Input: part model. Units: mm. Frame: model coordinates. A direction names the side the tool comes from. Round coordinates to 2 decimals unless told otherwise and drop trailing zeros. Loops run counter-clockwise (first coordinate to the right, second up) from the corner with the lowest first, then second, coordinate; pieces in that order, holes last. Notation, with made-up numbers: M 49,64 L 77,64 A25 ccw 77,76 Z; hole C 73.25,-23.5 d3. An arc over 180 degrees is marked long. Put each result on its own line as item: value. Start each with the question number.
1) Reachability of faces 5 (the face through (15, 5, 31.5)), 6 (the face through (-7, 14, 34.5)), 7 (the face through (0, 10, 0)) from +Z, -Z, +X, -X, +Y, -Y: full face, straight path, thin tool, end or side. Return the list, or none.
2) Section D-D on z = 37. Output: boundary loops of the cut face in (x, y), plus the area to 3 significant figures.
3) Line query: probe 1 along Z at (x, y) = (-7, 4.5); probe 2 along Y at (x, z) = (-7.08, 36.75); probe 3 along Z at (x, y) = (7.8, 2). Output: solid intervals per line, ascending.
4) Draft query along Z for faces 1 (the face through (-7, 10, 41.5)), 2 (the face through (-7, 20, 37)), 3 (the face through (8.421, 4.93, 15.797)), 4 (the face through (-7.487, 4.93, -16.954)). Return one class per face: +Z half, -Z half, draft (parallel to the pull), parting line (faces both ways), or undercut.
5) Pin query (flat end, axial travel): pin 1 (2.5 mm diameter, centred on x = -7, z = 23.5, fed in from -Y); pin 2 (1 mm diameter, centred on x = -11.5, z = 30, fed in from +Y); pin 3 (1.5 mm diameter, centred on x = 12.5, y = 5, fed in from +Z); pin 4 (8 mm diameter, centred on y = 3, z = 5, fed in from -X). Return the tip coordinate at first contact, or that it passes through.
6) Section B-B on z = 23.5. Output: boundary loops of the cut face in (x, y).
7) Section C-C on x = -11.5. Output: boundary loops of the cut face in (y, z), plus the area to 3 significant figures.
8) Section A-A on y = 4. Output: boundary loops of the cut face in (x, z), plus the area to 3 significant figures.
Autodesk Inventor part; units mm, degrees
ref_plane "YZ Plane" through (0, 0, 0) normal (1, 0, 0) x (0, 1, 0)
ref_plane "XZ Plane" through (0, 0, 0) normal (0, 1, 0) x (-1, 0, 0)
ref_plane "XY Plane" through (0, 0, 0) normal (0, 0, 1) x (1, 0, 0)
sketch "Sketch2" plane through (0, 0, 0) normal (0, 1, 0) x (-1, 0, 0)
  line L0 (0, -46.1) -> (0, 56.1)
  line L1 (33.556, 0) -> (-28.926, 0)
  line L2 (20, -31.5) -> (-20, -31.5)
  line L3 (-20, -31.5) -> (-20, 31.5)
  line L4 (-20, 31.5) -> (20, 31.5)
  line L5 (20, 31.5) -> (20, -31.5)
  line L6 (20, -31.5) -> (-20, 31.5) construction
  line L7 (-20, -31.5) -> (20, 31.5) construction
  line L8 (24.63, 31.5) -> (-10.47, 31.5)
  line L9 (-10.47, 31.5) -> (-10.47, 41.5)
  line L10 (-10.47, 41.5) -> (24.63, 41.5)
  line L11 (24.63, 41.5) -> (24.63, 31.5)
  line L12 (24.63, 31.5) -> (-10.47, 41.5) construction
  line L13 (-10.47, 31.5) -> (24.63, 41.5) construction
  point P0 (0, 0)
  point P1 (7.08, 36.5)
  point P2 (-10.47, 31.5)
  dimension "d5" = 40
  dimension "d6" = 63
  dimension "d7" = 9.53
  dimension "d8" = 35.1
  dimension "d9" = 73
extrude "Extrusion1" add sketch "Sketch2" along normal blind 10 contours L2 L3 L1 L0 | L0 L1 L5 L2 | L1 L3 L4 L0 | L0 L4 L5 L1
extrude "Extrusion2" add sketch "Sketch2" along normal blind 20 contours L4 L9 L10 L0 | L0 L10 L11 L8 L4
sketch "Sketch3" plane through (0, 10, 0) normal (0, 1, 0) x (1, 0, 0)
  line L0 (-20, 31.5) -> (-20, -31.5)
  line L1 (20, 31.5) -> (-20, 31.5)
  line L2 (20, -31.5) -> (20, 31.5)
  point P0 (0, 0)
  point P1 (-7, 18.5)
  point P2 (-7, -23.5)
  point P3 (7.8, 14.41)
  point P4 (7.8, -14.3)
  dimension "d21" = 13
  dimension "d22" = 13
  dimension "d23" = 42
  dimension "d24" = 13
  dimension "d25" = 12.2
  dimension "d26" = 12.2
  dimension "d27" = 17.09
  dimension "d28" = 28.71
hole "Hole1" at (-7, 10, -18.5) at (-7, 10, 23.5) at (7.8, 10, -14.41) at (7.8, 10, 14.3) direction (0, -1, 0) diameter 3.242 end through all
sketch "Sketch4" plane through (-24.63, 0, 41.5) normal (0, 0, 1) x (1, 0, 0)
  line L0 (0, 20) -> (35.1, 20)
  line L1 (35.1, 0) -> (35.1, 20)
  point P0 (24.63, 0)
  point P1 (17.55, 14.3)
  dimension "d36" = 5.7
  dimension "d37" = 17.55
hole "Hole2" at (-7.08, 14.3, 41.5) direction (0, 0, -1) diameter 7.4 depth 7
sketch "Sketch5" plane through (-24.63, 0, 41.5) normal (0, 0, 1) x (1, 0, 0)
  circle A0 centre (17.55, 14.3) radius 3.7
  line L0 (0, 0) -> (35.1, 0)
  line L1 (35.1, 0) -> (35.1, 20)
  point P0 (24.63, 0)
  point P1 (17.55, 4)
  dimension "d46" = 4
  dimension "d47" = 17.55
hole "Hole3" at (-7.08, 4, 41.5) direction (0, 0, -1) diameter 4 depth 7
properties part number "uchwyt_strzykawka_dol" material "PC/ABS Plastic"
Geometry results:
1. face 5: +Z, +X, +Y, -Y
1. face 6: +Z
1. face 7: -Z, +X, -X, +Y
2. outline: M -24.63,0 L 10.47,0 L 10.47,20 L -24.63,20 Z; hole C -7.08,14.3 d7.4; hole C -7.08,4 d4
2. area: 646 mm²
3. probe 1: z = -31.5 to -20.12, -16.88 to 21.88, 25.12 to 34.5
3. probe 2: y = 0 to 2, 6 to 10.6, 18 to 20
3. probe 3: z = -31.5 to -16.03, -12.79 to 12.68, 15.92 to 41.5
4. face 1: +Z half
4. face 2: draft
4. face 3: undercut
4. face 4: undercut
5. pin 1: passes through
5. pin 2: stops at y = 10
5. pin 3: stops at z = 31.5
5. pin 4: stops at x = -20
6. outline: M -20,0 L -8.62,0 L -8.62,10 L -20,10 Z; M -5.38,0 L 20,0 L 20,10 L -5.38,10 Z
7. outline: M 0,-31.5 L 10,-31.5 L 10,31.5 L 20,31.5 L 20,41.5 L 0,41.5 Z
7. area: 830 mm²
8. outline: M -24.63,31.5 L -20,31.5 L -20,-31.5 L 20,-31.5 L 20,31.5 L 10.47,31.5 L 10.47,41.5 L -5.08,41.5 L -5.08,34.5 L -9.08,34.5 L -9.08,41.5 L -24.63,41.5 Z; hole C -7,-18.5 d3.24; hole C -7,23.5 d3.24; hole C 7.8,-14.41 d3.24; hole C 7.8,14.3 d3.24
8. area: 2,810 mm²
